Autodesk Inventor part; units mm, degrees
ref_plane "YZ Plane" through (0, 0, 0) normal (1, 0, 0) x (0, 1, 0)
ref_plane "XZ Plane" through (0, 0, 0) normal (0, 1, 0) x (-1, 0, 0)
ref_plane "XY Plane" through (0, 0, 0) normal (0, 0, 1) x (1, 0, 0)
sketch "Sketch2" plane through (0, 0, 0) normal (0, 0, 1) x (1, 0, 0)
  line L0 (-9.25, -9.5) -> (9.25, -9.5)
  line L1 (9.5, -9.25) -> (9.5, 9.25)
  line L2 (9.25, 9.5) -> (-9.25, 9.5)
  line L3 (-9.5, 9.25) -> (-9.5, -9.25)
  line L4 (-9.5, -9.5) -> (9.5, 9.5) construction
  line L5 (9.5, -9.5) -> (-9.5, 9.5) construction
  line L6 (-7.65, 7.9) -> (7.65, 7.9)
  line L7 (7.9, 7.65) -> (7.9, -7.65)
  line L8 (7.65, -7.9) -> (-7.65, -7.9)
  line L9 (-7.9, -7.65) -> (-7.9, 7.65)
  arc A0 (-9.25, 9.5) -> (-9.5, 9.25) centre (-9.25, 9.25) ccw
  arc A1 (-7.65, 7.9) -> (-7.9, 7.65) centre (-7.65, 7.65) ccw
  arc A2 (9.5, 9.25) -> (9.25, 9.5) centre (9.25, 9.25) ccw
  arc A3 (9.25, -9.5) -> (9.5, -9.25) centre (9.25, -9.25) ccw
  arc A4 (-9.5, -9.25) -> (-9.25, -9.5) centre (-9.25, -9.25) ccw
  arc A5 (-7.9, -7.65) -> (-7.65, -7.9) centre (-7.65, -7.65) ccw
  arc A6 (7.9, 7.65) -> (7.65, 7.9) centre (7.65, 7.65) ccw
  arc A7 (7.65, -7.9) -> (7.9, -7.65) centre (7.65, -7.65) ccw
  point P0 (0, 0)
  dimension "d0" = 19
  dimension "d1" = 19
  dimension "d2" = 1.6
  dimension "d3" = 0.25
extrude "Extrusion1" add sketch "Sketch2" against normal blind 760
sketch "Sketch3" plane through (-9.25, -9.5, 0) normal (0, -1, 0) x (1, 0, 0)
  circle A0 centre (9.25, -713.9463) radius 3.175
  circle A1 centre (9.25, -563.9463) radius 3.175
  point P0 (9.25, 0)
hole "Hole1" at (0, -9.5, -563.9463) at (0, -9.5, -713.9463) direction (0, 1, 0) diameter 5.5 end through all
sketch "Sketch5" plane through (-9.25, -9.5, 0) normal (0, -1, 0) x (1, 0, 0)
  circle A0 centre (9.25, -375.6475) radius 3
  point P0 (9.25, 0)
hole "Hole2" at (0, -9.5, -375.6475) direction (0, 1, 0) diameter 6 end through all
properties part number "bpSupArm37"
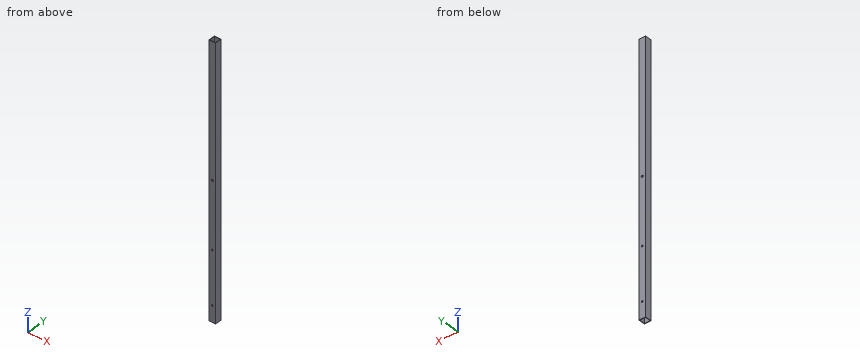
Source: CAD feature listing. Evaluate the final solid. Frame: model axes, mm. Round coordinates to 2 decimals unless told otherwise and drop trailing zeros. Loops run counter-clockwise (first coordinate to the right, second up) from the corner with the lowest first, then second, coordinate; pieces in that order, holes last. Notation, with made-up numbers: (17, -9) -> (59, -9) arc R21 cw to (59, 22) -> close; hole circle Ø8 at (-11.75, 83.25). An arc over 180 degrees is marked (long way). Answer as a JSON object with one key per item and string values. Group by question number.
Q1. Ray query, line 1 (X direction, y = 1, z = -328); line 2 (Z direction, x = 0, y = -8.6). Return the intervals inside material, ascending. Write a range as from..to.
Q2. Section query B-B (z = -473). Output: boundary loops of the cut face in (x, y).
Q3. Contact query for a flat-ended pin moving along its axis: P1, Ø5, axis at x = 0, z = -563.95, coming from the -Y side. Output: stop coordinate, or through.
Q4. Section query A-A (y = 3.5). Output: boundary loops of the cut face in (x, z).
Completed:
{
 "1": {"line 1": "-9.5..-7.9, 7.9..9.5", "line 2": "-760..-716.7, -711.2..-566.7, -561.2..-378.65, -372.65..0"},
 "2": {"outline": "(-9.5, -9.25) arc R0.25 ccw to (-9.25, -9.5) -> (9.25, -9.5) arc R0.25 ccw to (9.5, -9.25) -> (9.5, 9.25) arc R0.25 ccw to (9.25, 9.5) -> (-9.25, 9.5) arc R0.25 ccw to (-9.5, 9.25) -> close; hole (-7.9, -7.65) arc R0.25 ccw to (-7.65, -7.9) -> (7.65, -7.9) arc R0.25 ccw to (7.9, -7.65) -> (7.9, 7.65) arc R0.25 ccw to (7.65, 7.9) -> (-7.65, 7.9) arc R0.25 ccw to (-7.9, 7.65) -> close"},
 "3": {"P1": "through"},
 "4": {"outline": "(-9.5, -760) -> (-7.9, -760) -> (-7.9, 0) -> (-9.5, 0) -> close; (7.9, -760) -> (9.5, -760) -> (9.5, 0) -> (7.9, 0) -> close"}
}
